Geometry check sheet. Reference: the model listing, model coordinates, mm. A direction names the side the tool comes from. Round coordinates to 2 decimals unless told otherwise and drop trailing zeros. Write each loop counter-clockwise with the first axis right and the second up, starting at its lowest first coordinate (ties: lowest second). Pieces come first, ordered by that corner, then holes. Notation, with made-up numbers: (51.25, 27) -> (60.25, 27) arc R13 cw to (60.25, 44) -> close; hole circle Ø4 at (-20.5, 31). An arc over 180 degrees is marked (long way). Return JSON: item names as keys, results as strings. Group by question number.
from build123d import *

# Parameters (mm, degrees)
EXTRUDE_1_DEPTH                  = 1
SM_EDGE_FLANGE_1_STRIP_W         = 6
SM_EDGE_FLANGE_1_STRIP_H         = 1
SM_EDGE_FLANGE_1_STRIP_CUT_DEPTH = 410
SM_EDGE_FLANGE_1_DEPTH           = 410


# Sheet-metal steps are written as plain solids
with BuildPart() as part:
    # Sketch 1 → Бобышка-Вытянуть1 (new body)
    with BuildSketch(Plane(origin=(0, 0, 0), x_dir=(0, 0, -1), z_dir=(1, 0, 0))):
        Polygon((-262, -165), (262, -165), (262, -35), (148, 130), (148, 165), (-262, 165), align=None)
    extrude(amount=EXTRUDE_1_DEPTH)

    # Ребро-кромка1 strip (across the edge) → Ребро-кромка1 strip cut (cut)
    with BuildSketch(Plane(origin=(1, 165, -148), x_dir=(0, -1, 0), z_dir=(0, 0, 1))):
        with Locations((-1, -0.5)):
            Rectangle(SM_EDGE_FLANGE_1_STRIP_W, SM_EDGE_FLANGE_1_STRIP_H)
    extrude(amount=SM_EDGE_FLANGE_1_STRIP_CUT_DEPTH, mode=Mode.SUBTRACT)

    # Ребро-кромка1 section (across the edge) → Ребро-кромка1 (add)
    with BuildSketch(Plane(origin=(1, 165, -148), x_dir=(0, -1, 0), z_dir=(0, 0, 1))):
        with BuildLine():
            Line((0, 1), (0, 49))
            Line((0, 49), (1, 49))
            Line((1, 49), (1, 1))
            ThreePointArc((1, 1), (1.292893219, 0.292893219), (2, 0))
            Line((2, 0), (2, -1))
            ThreePointArc((2, -1), (0.585786438, -0.414213562), (0, 1))
        make_face()
    extrude(amount=SM_EDGE_FLANGE_1_DEPTH)


solid = part.part
1) Sectioned sample at A-A on z = -110.5. Enter the section's corners in (x, y).
2) Tool access check on faces 1 (the face through (1, 1, 4)), 2 (the face through (0, 1, 4)). Record the directions out of +Z, -Z, +X, -X, +Y, -Y that give a thin tool (end or side, any length) a straight path to the whole face; none if there is none.
3) Sectioned sample at C-C on x = 17. Enter the section's corners in (y, z).
4) Sectioned sample at B-B on y = -76. Enter the section's corners in (x, z), and give its area (3 significant figures).
5) Go/stop test with flat-tipped pins: P1, Ø8, axis at y = -116.5, z = -152.5, coming from the +X side; P2, Ø2, axis at x = 35.5, z = 199.5, coming from the -Y side. Record where each tip stops, or that it passes through.
6) Material ranges on probe 1 along X at (y, z) = (138, -48); probe 2 along Y at (x, z) = (31, -14), recorded low to high. Write a range as [from, to].
Evaluation:
{
 "1": {"outline": "(0, -165) -> (1, -165) -> (1, 163) arc R1 cw to (2, 164) -> (50, 164) -> (50, 165) -> (2, 165) arc R2 ccw to (0, 163) -> close"},
 "2": {"face 1": "+Z, -Z, +X, -Y", "face 2": "+Z, -Z, -X, +Y, -Y"},
 "3": {"outline": "(164, -148) -> (165, -148) -> (165, 262) -> (164, 262) -> close"},
 "4": {"outline": "(0, -262) -> (1, -262) -> (1, 262) -> (0, 262) -> close", "area": "524 mm2"},
 "5": {"P1": "stops at x = 1", "P2": "stops at y = 164"},
 "6": {"probe 1": "x = [0, 1]", "probe 2": "y = [164, 165]"}
}
